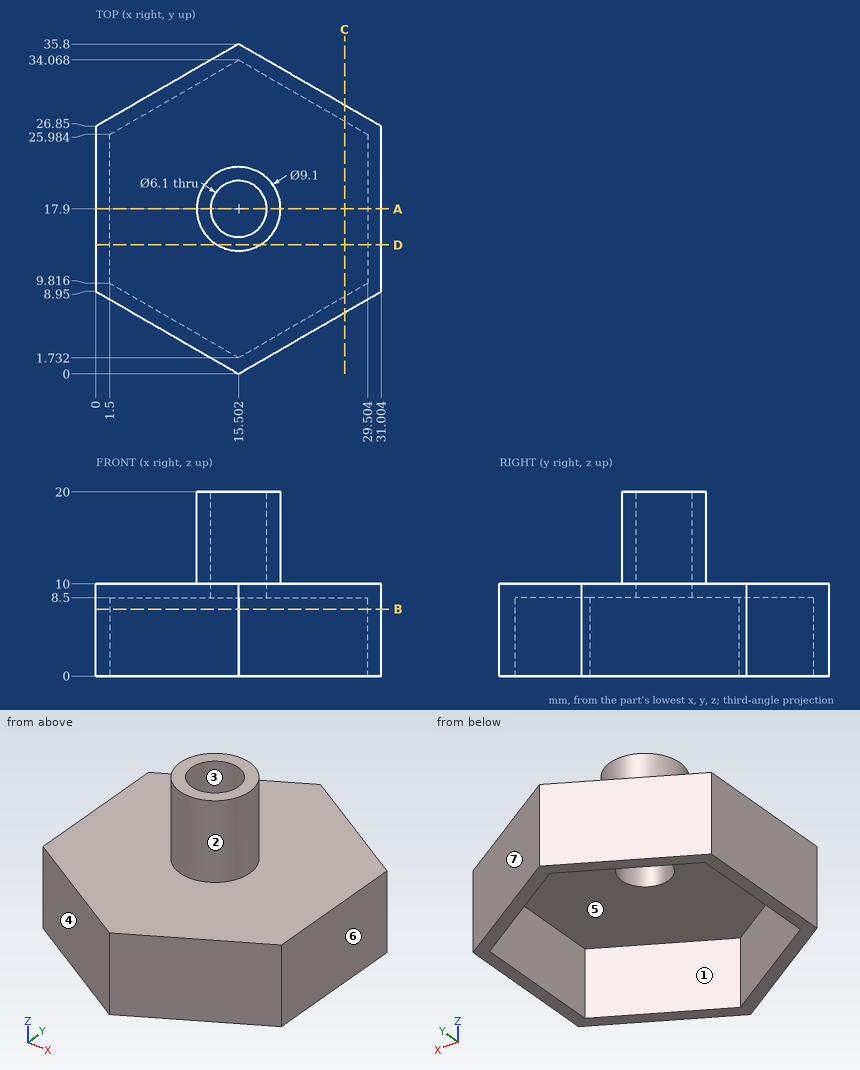
For this review, use the dimensioned drawing (mm, ordinates from the lowest corner) and the shaded views. A direction names the side the tool comes from. Round coordinates to 2 decimals unless told otherwise and drop trailing zeros. Order: outer loops, then holes, each group sorted by start corner. A loop starts at its lowest first (then second) coordinate and runs counter-clockwise, first axis right, second up. Notation, with made-up numbers: M 75.5,48 L 79.5,48 A21 cw 79.5,70 Z; hole C 21,33.25 d7. An arc over 180 degrees is marked long. Use a Markdown table: item, result.
1) Consider section C-C (x = 27). Write out the cut boundary in (y, z).
Report:
| item | result |
|---|---|
| outline | M 6.64,0 L 8.37,0 L 8.37,8.5 L 27.43,8.5 L 27.43,0 L 29.16,0 L 29.16,10 L 6.64,10 Z |
2) Insertion check: pin 1 (5 mm diameter, centred on x = 10, z = 13.5, fed in from -Y); pin 2 (5 mm diameter, centred on x = 7, y = 15, fed in from -Z); pin 3 (2 mm diameter, centred on y = 16, z = 12.5, fed in from +X). Each pin has a flat end and moves straight along its axis. Give the tip position at first contact, or say it passes through.
Report:
| item | result |
|---|---|
| pin 1 | y = 14.48 |
| pin 2 | z = 8.5 |
| pin 3 | x = 19.96 |
3) Consider section B-B (z = 7.25). Write out the cut boundary in (x, y), then the cut area to 3 significant figures.
Report:
| item | result |
|---|---|
| outline | M 0,8.95 L 15.5,0 L 31,8.95 L 31,26.85 L 15.5,35.8 L 0,26.85 Z; hole M 1.5,9.82 L 15.5,1.73 L 29.5,9.82 L 29.5,25.98 L 15.5,34.07 L 1.5,25.98 Z |
| area | 153 mm^2 |
4) Wall thickness on line 1 along X through (y, z) = (20.5, 2); line 2 along Z through (x, y) = (7, 28); line 3 along Y through (x, z) = (13.5, 3.5) (1 decimal): over which ranges is each line inside the solid? List them lowest first. Write a range as [from, to].
Report:
| item | result |
|---|---|
| line 1 | [0, 1.5], [29.5, 31] |
| line 2 | [8.5, 10] |
| line 3 | [1.2, 2.9], [32.9, 34.6] |
5) Draft analysis for pull direction Y (two halves, no side actions). For the marked faces 4, 5, 6 and 7, state which applies: released by +Y, released by -Y, zero draft, split by the parting line, or undercut.
Report:
| item | result |
|---|---|
| face 4 | released by -Y |
| face 5 | undercut |
| face 6 | zero draft |
| face 7 | released by +Y |
6) Consider section D-D (y = 14). Write out the cut boundary in (x, z) (1 decimal), then the cut area to 3 significant figures.
Report:
| item | result |
|---|---|
| outline | M 0,0 L 1.5,0 L 1.5,8.5 L 29.5,8.5 L 29.5,0 L 31,0 L 31,10 L 17.8,10 L 17.8,20 L 13.2,20 L 13.2,10 L 0,10 Z |
| area | 119 mm^2 |
7) Consider section A-A (y = 17.9). Write out the cut boundary in (x, z).
Report:
| item | result |
|---|---|
| outline | M 0,0 L 1.5,0 L 1.5,8.5 L 12.45,8.5 L 12.45,20 L 10.95,20 L 10.95,10 L 0,10 Z; M 18.55,8.5 L 29.5,8.5 L 29.5,0 L 31,0 L 31,10 L 20.05,10 L 20.05,20 L 18.55,20 Z |
8) Tool access review of the marked faces 1, 2 and 3: name each direction out of +Z, -Z, +X, -X, +Y, -Y from which nothing blocks a thin tool from reaching the whole face with its end or side.
Report:
| item | result |
|---|---|
| face 1 | -Z |
| face 2 | +Z |
| face 3 | +Z, -Z |
